from build123d import *

# Parameters (mm, degrees)
F1_DEPTH = 25
F2_W     = 3
F2_H     = 9
F4_R     = 1.5
F5_DEPTH = 10.0385235668


with BuildPart() as f1:
    # F0 (on Front) → F1 (new body)
    with BuildSketch(Plane.XZ):
        with BuildLine():
            Line((0, 250), (0, 0))
            ThreePointArc((0, 0), (40, -40), (80, 0))
            Line((80, 0), (80, 250))
            ThreePointArc((80, 250), (40, 290), (0, 250))
        make_face()
        with BuildLine():
            ThreePointArc((10, 250), (40, 280), (70, 250))
            Line((70, 250), (70, 0))
            ThreePointArc((70, 0), (40, -30), (10, 0))
            Line((10, 0), (10, 250))
        make_face(mode=Mode.SUBTRACT)
    extrude(amount=F1_DEPTH)

    # F3: sweep along a path in F3_path
    with BuildLine(Plane(origin=(10, -25, 0), x_dir=(0, 0, -1), z_dir=(0, 1, 0))) as f3_path:
        Line((0, 0), (-250, 0))
        ThreePointArc((-250, 0), (-280, -30), (-250, -60))
        Line((-250, -60), (0, -60))
    # F2 (on Top) → F3 (sweep, cut)
    with BuildSketch(Plane.XY):
        with Locations((8.5, -12.5)):
            Rectangle(F2_W, F2_H)
    sweep(path=f3_path.line, mode=Mode.SUBTRACT)

    # F4 (on face) → F5 (cut, through all)
    with BuildSketch(Plane.YZ.offset(80)):
        with Locations((-12.5, 0)):
            Circle(F4_R)
    extrude(amount=-F5_DEPTH, mode=Mode.SUBTRACT)


solid = f1.part
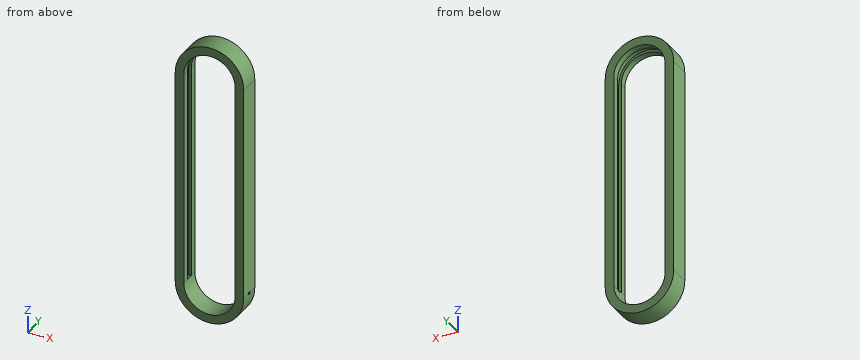
Read the model definition and answer for the solid it produces. Units are mm, in the model's axes. Coordinates: 2 decimals unless noted, no trailing zeros. Loops run counter-clockwise (first coordinate to the right, second up) from the corner with the lowest first, then second, coordinate; pieces in that order, holes last.
Q1. The part is cut by section D-D on x = 19.5. Write down the section's boundary in (y, z), and give its area (3 significant figures).
Q2. The part is cut by section C-C on y = -4.25. Write down the section's boundary in (x, z), and give its area (3 significant figures).
Q3. The part is cut by section B-B on z = 60.5. Write down the section's boundary in (x, y).
Q4. The part is cut by section A-A on x = 40. Write down the section's boundary in (y, z).
Q5. Each of these flat-tipped pins is pushed along its axis until it touches: pin 1 Ø4 at (y, z) = (-21.5, 115) entering from -X; pin 2 Ø0.9 at (x, y) = (8.5, -12.5) entering from +Z; pin 3 Ø1.5 at (x, y) = (71.5, -10) entering from +Z; pin 4 Ø3.5 at (x, y) = (72, -15.5) entering from +Z. Where does it stop, or does it pass through?
Q6. Consider probe 1 along X at (y, z) = (-12.75, 144.5); probe 2 along X at (y, z) = (-2.25, 103.5); probe 3 along Z at (x, y) = (38.5, -11). Determine where each line is inside the solid, lowest interval first.
Results below:
1. outline: (-25, -34.35) - (0, -34.35) - (0, -21.9) - (-25, -21.9) - close; (-25, 271.9) - (-17, 271.9) - (-17, 275.86) - (-8, 275.86) - (-8, 271.9) - (0, 271.9) - (0, 284.35) - (-25, 284.35) - close
1. area: 587 mm2
2. outline: (0, 0) arc R40 ccw to (80, 0) - (80, 250) arc R40 ccw to (0, 250) - close; hole (10, 0) arc R30 ccw to (70, 0) - (70, 250) arc R30 ccw to (10, 250) - close
2. area: 7,200 mm2
3. outline: (0, -25) - (10, -25) - (10, -17) - (7, -17) - (7, -8) - (10, -8) - (10, 0) - (0, 0) - close; (70, -25) - (80, -25) - (80, 0) - (70, 0) - (70, -8) - (73, -8) - (73, -17) - (70, -17) - close
4. outline: (-25, -40) - (0, -40) - (0, -30) - (-25, -30) - close; (-25, 280) - (-17, 280) - (-17, 283) - (-8, 283) - (-8, 280) - (0, 280) - (0, 290) - (-25, 290) - close
5. pin 1: stops at x = 0
5. pin 2: stops at z = 275.22
5. pin 3: stops at z = 275.58
5. pin 4: stops at z = 276.17
6. probe 1: x = 0 to 7, 73 to 80
6. probe 2: x = 0 to 10, 70 to 80
6. probe 3: z = -39.97 to -29.96, 282.97 to 289.97
